from build123d import *

# Parameters (mm, degrees)
CYLINDER2682_R               = 1.5
CYLINDER2682_DEPTH           = 60
CYLINDER2681_R               = 1.5
CYLINDER2681_DEPTH           = 60
TUBE120_R                    = 31
TUBE120_R_2                  = 22
TUBE120_DEPTH                = 24
CYLINDER2647_R               = 14
CYLINDER2647_DEPTH           = 5
CYLINDER2632_R               = 1.5
CYLINDER2632_DEPTH           = 20
CYLINDER2632_PLACEMENT_ANGLE = 45
CYLINDER2640_R               = 1.5
CYLINDER2640_DEPTH           = 20
CYLINDER2633_R               = 1.5
CYLINDER2633_DEPTH           = 20
CYLINDER2633_PLACEMENT_ANGLE = 135
CYLINDER2641_R               = 1.5
CYLINDER2641_DEPTH           = 20
CYLINDER2634_R               = 1.5
CYLINDER2634_DEPTH           = 20
CYLINDER2634_PLACEMENT_ANGLE = 225
CYLINDER2644_R               = 1.5
CYLINDER2644_DEPTH           = 20
CYLINDER2643_R               = 1.5
CYLINDER2643_DEPTH           = 20
CYLINDER2643_PLACEMENT_ANGLE = 45
CYLINDER2646_R               = 1.5
CYLINDER2646_DEPTH           = 20
CYLINDER2635_R               = 3
CYLINDER2635_DEPTH           = 3
CYLINDER2635_PLACEMENT_ANGLE = 45
CYLINDER2636_R               = 3
CYLINDER2636_DEPTH           = 3
CYLINDER2630_R               = 3
CYLINDER2630_DEPTH           = 3
CYLINDER2630_PLACEMENT_ANGLE = 135
CYLINDER2631_R               = 3
CYLINDER2631_DEPTH           = 5
CYLINDER2637_R               = 3
CYLINDER2637_DEPTH           = 5
CYLINDER2637_PLACEMENT_ANGLE = 225
CYLINDER2638_R               = 3
CYLINDER2638_DEPTH           = 3
CYLINDER2639_R               = 3
CYLINDER2639_DEPTH           = 3
CYLINDER2639_PLACEMENT_ANGLE = 45
CYLINDER2642_R               = 3
CYLINDER2642_DEPTH           = 3
CYLINDER2645_R               = 38
CYLINDER2645_DEPTH           = 6
CHAMFER126_SIZE              = 1
CHAMFER126_ROLL_ANGLE        = 180
CHAMFER126_PLACEMENT_ANGLE   = -157.5


with BuildPart() as obj1:
    # Cylinder2682 → Cylinder2682 (new body)
    with BuildSketch(Plane(origin=(33, -10, 8), x_dir=(1, 0, 0), z_dir=(0, -1, 0))):
        Circle(CYLINDER2682_R)
    extrude(amount=CYLINDER2682_DEPTH)


with BuildPart() as compound1193:
    # Cylinder2681 → Cylinder2681 (new body)
    with BuildSketch(Plane(origin=(-33, -10, 8), x_dir=(1, 0, 0), z_dir=(0, -1, 0))):
        Circle(CYLINDER2681_R)
    extrude(amount=CYLINDER2681_DEPTH)

    # Compound1193: union obj1
    add(obj1.part)


with BuildPart() as compound1193_1:
    # Compound1193 placement: moved
    add(compound1193.part.moved(Location((0, -1, 0))))


with BuildPart() as tube120:
    # Tube120 → Tube120 (new body)
    with BuildSketch(Plane(origin=(0, -17, 37), x_dir=(1, 0, 0), z_dir=(0, -1, 0))):
        Circle(TUBE120_R)
        Circle(TUBE120_R_2, mode=Mode.SUBTRACT)
    extrude(amount=TUBE120_DEPTH)


with BuildPart() as obj2:
    # Cylinder2647 → Cylinder2647 (new body)
    with BuildSketch(Plane.XY.offset(1)):
        Circle(CYLINDER2647_R)
    extrude(amount=CYLINDER2647_DEPTH)


with BuildPart() as obj3:
    # Cylinder2632 → Cylinder2632 (new body)
    with BuildSketch(Plane.XY):
        Circle(CYLINDER2632_R)
    extrude(amount=CYLINDER2632_DEPTH)


with BuildPart() as obj3_1:
    # Cylinder2632 placement: moved
    add(obj3.part.moved(Location((-19.445436, 19.445436, 19))).rotate(Axis((-19.445436, 19.445436, 19), (0, 0, 1)), CYLINDER2632_PLACEMENT_ANGLE))


with BuildPart() as obj4:
    # Cylinder2640 → Cylinder2640 (new body)
    with BuildSketch(Plane(origin=(-27.5, 0, 19), x_dir=(0, 1, 0), z_dir=(0, 0, 1))):
        Circle(CYLINDER2640_R)
    extrude(amount=CYLINDER2640_DEPTH)


with BuildPart() as obj5:
    # Cylinder2633 → Cylinder2633 (new body)
    with BuildSketch(Plane.XY):
        Circle(CYLINDER2633_R)
    extrude(amount=CYLINDER2633_DEPTH)


with BuildPart() as obj5_1:
    # Cylinder2633 placement: moved
    add(obj5.part.moved(Location((-19.445436, -19.445436, 19))).rotate(Axis((-19.445436, -19.445436, 19), (0, 0, 1)), CYLINDER2633_PLACEMENT_ANGLE))


with BuildPart() as obj6:
    # Cylinder2641 → Cylinder2641 (new body)
    with BuildSketch(Plane(origin=(0, -27.5, 19), x_dir=(-1, 0, 0), z_dir=(0, 0, 1))):
        Circle(CYLINDER2641_R)
    extrude(amount=CYLINDER2641_DEPTH)


with BuildPart() as obj7:
    # Cylinder2634 → Cylinder2634 (new body)
    with BuildSketch(Plane.XY):
        Circle(CYLINDER2634_R)
    extrude(amount=CYLINDER2634_DEPTH)


with BuildPart() as obj7_1:
    # Cylinder2634 placement: moved
    add(obj7.part.moved(Location((19.445436, -19.445436, 19))).rotate(Axis((19.445436, -19.445436, 19), (0, 0, 1)), CYLINDER2634_PLACEMENT_ANGLE))


with BuildPart() as obj8:
    # Cylinder2644 → Cylinder2644 (new body)
    with BuildSketch(Plane(origin=(27.5, 0, 19), x_dir=(0, -1, 0), z_dir=(0, 0, 1))):
        Circle(CYLINDER2644_R)
    extrude(amount=CYLINDER2644_DEPTH)


with BuildPart() as obj9:
    # Cylinder2643 → Cylinder2643 (new body)
    with BuildSketch(Plane.XY):
        Circle(CYLINDER2643_R)
    extrude(amount=CYLINDER2643_DEPTH)


with BuildPart() as obj9_1:
    # Cylinder2643 placement: moved
    add(obj9.part.moved(Location((19.445436, 19.445436, 19))).rotate(Axis((19.445436, 19.445436, 19), (0, 0, -1)), CYLINDER2643_PLACEMENT_ANGLE))


with BuildPart() as compound1169:
    # Cylinder2646 → Cylinder2646 (new body)
    with BuildSketch(Plane(origin=(0, 27.5, 19), x_dir=(1, 0, 0), z_dir=(0, 0, 1))):
        Circle(CYLINDER2646_R)
    extrude(amount=CYLINDER2646_DEPTH)

    # Compound1169: union obj3, obj4, obj5, obj6, obj7, obj8, obj9
    add(obj3_1.part)
    add(obj4.part)
    add(obj5_1.part)
    add(obj6.part)
    add(obj7_1.part)
    add(obj8.part)
    add(obj9_1.part)


with BuildPart() as compound1169_1:
    # Compound1169 placement: moved
    add(compound1169.part.moved(Location((0, 0, -23))))


with BuildPart() as obj10:
    # Cylinder2635 → Cylinder2635 (new body)
    with BuildSketch(Plane.XY):
        Circle(CYLINDER2635_R)
    extrude(amount=CYLINDER2635_DEPTH)


with BuildPart() as obj10_1:
    # Cylinder2635 placement: moved
    add(obj10.part.moved(Location((-19.45, 19.45, 19))).rotate(Axis((-19.45, 19.45, 19), (0, 0, 1)), CYLINDER2635_PLACEMENT_ANGLE))


with BuildPart() as obj11:
    # Cylinder2636 → Cylinder2636 (new body)
    with BuildSketch(Plane(origin=(-27.5, 0, 19), x_dir=(0, 1, 0), z_dir=(0, 0, 1))):
        Circle(CYLINDER2636_R)
    extrude(amount=CYLINDER2636_DEPTH)


with BuildPart() as obj12:
    # Cylinder2630 → Cylinder2630 (new body)
    with BuildSketch(Plane.XY):
        Circle(CYLINDER2630_R)
    extrude(amount=CYLINDER2630_DEPTH)


with BuildPart() as obj12_1:
    # Cylinder2630 placement: moved
    add(obj12.part.moved(Location((-19.445436, -19.445436, 19))).rotate(Axis((-19.445436, -19.445436, 19), (0, 0, 1)), CYLINDER2630_PLACEMENT_ANGLE))


with BuildPart() as obj13:
    # Cylinder2631 → Cylinder2631 (new body)
    with BuildSketch(Plane(origin=(0, -27.5, 19.5), x_dir=(-1, 0, 0), z_dir=(0, 0, 1))):
        Circle(CYLINDER2631_R)
    extrude(amount=CYLINDER2631_DEPTH)


with BuildPart() as obj14:
    # Cylinder2637 → Cylinder2637 (new body)
    with BuildSketch(Plane.XY):
        Circle(CYLINDER2637_R)
    extrude(amount=CYLINDER2637_DEPTH)


with BuildPart() as obj14_1:
    # Cylinder2637 placement: moved
    add(obj14.part.moved(Location((19.45, -19.45, 19.5))).rotate(Axis((19.45, -19.45, 19.5), (0, 0, 1)), CYLINDER2637_PLACEMENT_ANGLE))


with BuildPart() as obj15:
    # Cylinder2638 → Cylinder2638 (new body)
    with BuildSketch(Plane(origin=(27.5, 0, 19), x_dir=(0, -1, 0), z_dir=(0, 0, 1))):
        Circle(CYLINDER2638_R)
    extrude(amount=CYLINDER2638_DEPTH)


with BuildPart() as obj16:
    # Cylinder2639 → Cylinder2639 (new body)
    with BuildSketch(Plane.XY):
        Circle(CYLINDER2639_R)
    extrude(amount=CYLINDER2639_DEPTH)


with BuildPart() as obj16_1:
    # Cylinder2639 placement: moved
    add(obj16.part.moved(Location((19.445436, 19.445436, 19))).rotate(Axis((19.445436, 19.445436, 19), (0, 0, -1)), CYLINDER2639_PLACEMENT_ANGLE))


with BuildPart() as compound1170:
    # Cylinder2642 → Cylinder2642 (new body)
    with BuildSketch(Plane(origin=(0, 27.5, 19), x_dir=(1, 0, 0), z_dir=(0, 0, 1))):
        Circle(CYLINDER2642_R)
    extrude(amount=CYLINDER2642_DEPTH)

    # Compound1170: union obj10, obj11, obj12, obj13, obj14, obj15, obj16
    add(obj10_1.part)
    add(obj11.part)
    add(obj12_1.part)
    add(obj13.part)
    add(obj14_1.part)
    add(obj15.part)
    add(obj16_1.part)


with BuildPart() as compound1170_1:
    # Compound1170 placement: moved
    add(compound1170.part.moved(Location((0, 0, -19))))


with BuildPart() as cut1006:
    # Cylinder2645 → Cylinder2645 (new body)
    with BuildSketch(Plane.XY):
        Circle(CYLINDER2645_R)
    extrude(amount=CYLINDER2645_DEPTH)

    # Cut630: cut Compound1170
    add(compound1170_1.part, mode=Mode.SUBTRACT)

    # Cut628: cut Compound1169
    add(compound1169_1.part, mode=Mode.SUBTRACT)

    # Cut629: cut obj2
    add(obj2.part, mode=Mode.SUBTRACT)

    # Chamfer126
    chamfer126_edges = [cut1006.edges().sort_by_distance(p)[0] for p in [
        (-38, 0, 0),
    ]]
    chamfer(chamfer126_edges, length=CHAMFER126_SIZE)


with BuildPart() as cut1006_1:
    # Chamfer126 roll: moved
    add(cut1006.part.rotate(Axis((0, 0, 0), (1, 0, 0)), CHAMFER126_ROLL_ANGLE))


with BuildPart() as cut1006_2:
    # Chamfer126 placement: moved
    add(cut1006_1.part.moved(Location((0, 0, 11))).rotate(Axis((0, 0, 11), (0, 0, 1)), CHAMFER126_PLACEMENT_ANGLE))

    # Cut976: cut Tube120
    add(tube120.part, mode=Mode.SUBTRACT)

    # Cut1006: cut Compound1193
    add(compound1193_1.part, mode=Mode.SUBTRACT)


solid = cut1006_2.part
For this review, take the finished solid that the model builds, in its own axes (mm). A direction names the side the tool comes from. Round coordinates to 2 decimals unless told otherwise and drop trailing zeros. Write each loop counter-clockwise with the first axis right and the second up, starting at its lowest first coordinate (ties: lowest second). Pieces come first, ordered by that corner, then holes. Notation, with made-up numbers: (77.25, 81.5) - (91.25, 81.5) arc R26 ccw to (91.25, 111.5) - close; hole circle Ø5 at (6, -25.5). An arc over 180 degrees is marked (long way). Use a Markdown table: item, result.
Q1. Wall thickness on line 1 along X through (y, z) = (10.5, 10.5); line 2 along Y through (x, z) = (-11, 9.5); line 3 along X through (y, z) = (24.5, 8.5): over which ranges is each line inside the solid? List them lowest first.
Derived:
| item | result |
|---|---|
| line 1 | x = -36 to -28.41, -22.41 to 22.41, 28.41 to 36 |
| line 2 | y = -17 to -8.66, 8.66 to 22.44, 28.37 to 36.37 |
| line 3 | x = -29.05 to -13.38, -7.66 to 7.67, 13.38 to 29.05 |
Q2. Machinability: for faces 1 (the flat face through (0, 0, 10)), 2 (the cylindrical face through (0, -27, 6)), 3 (the cylindrical face through (-13.345, -26.44, 6.936)), 4 (the flat face through (-33, -11, 8)), which of the approach directions +Z, -Z, +X, -X, +Y, -Y give a long, thin tool a straight path to every point of the face, cutting with its end or side? Answer none if there is none.
Derived:
| item | result |
|---|---|
| face 1 | -Z |
| face 2 | +Z, -Y |
| face 3 | +Z |
| face 4 | -Y |
Q3. The part is to be moulded in two halves that separate along Z. For faces 5 (the cylindrical face through (28.36, -10, 9.52)), 6 (the flat face through (-10, 27, 8)), 7 (the cylindrical face through (31.5, -14.92, 8.07)), say which applies: pulls with the +Z half, pulls with the -Z half, needs draft (parallel to the pull), parting line crosses it, or undercut.
Derived:
| item | result |
|---|---|
| face 5 | needs draft |
| face 6 | pulls with the +Z half |
| face 7 | undercut |
Q4. Clearance check with flat-ended pins moving along their axes: pin 1 (2.5 mm diameter, centred on x = 25.41, y = 10.52, fed in from +Z); pin 2 (3.5 mm diameter, centred on x = -10.53, y = -25.41, fed in from +Z); pin 3 (1.5 mm diameter, centred on x = 27, z = 7, fed in from -Y); pin 4 (1 mm diameter, centred on x = 10.5, z = 9.5, fed in from -Y). State where each tip first meets the part, or that it passes through.
Derived:
| item | result |
|---|---|
| pin 1 | passes through |
| pin 2 | stops at z = 5.5 |
| pin 3 | stops at y = -27.48 |
| pin 4 | stops at y = -17 |
Q5. We need section B-B (x = 0). Give the boundary of the cut face in (y, z).
Derived:
| item | result |
|---|---|
| outline | (-38, 5) - (-14, 5) - (-14, 10) - (14, 10) - (14, 5) - (38, 5) - (38, 10) - (37, 11) - (-17, 11) - (-17, 6) - (-38, 6) - close |
Q6. We need section A-A (y = 0). Give the boundary of the cut face in (x, z), plus the area to 3 significant figures.
Derived:
| item | result |
|---|---|
| outline | (-38, 5) - (-14, 5) - (-14, 10) - (14, 10) - (14, 5) - (38, 5) - (38, 10) - (37, 11) - (-37, 11) - (-38, 10) - close |
| area | 315 mm2 |
